The model under review builds one solid part; all positions refer to its coordinate system, in mm. A direction names the side the tool comes from. Round coordinates to 2 decimals unless told otherwise and drop trailing zeros. Order: outer loops, then holes, each group sorted by start corner. A loop starts at its lowest first (then second) coordinate and runs counter-clockwise, first axis right, second up.
from build123d import *

# Parameters (mm, degrees)
F0_W     = 101.6
F0_H     = 101.6
F1_DEPTH = 101.6
F2_T     = -12.7
F3_W     = 12.7
F3_H     = 76.2
F4_DEPTH = 6.35
F5_R     = 2.54
F6_DEPTH = 95.885
F7_R     = 5.08


with BuildPart() as f1:
    # F0 (on Top) → F1 (new body)
    with BuildSketch(Plane.XY):
        Rectangle(F0_W, F0_H)
    extrude(amount=F1_DEPTH)

    # F2
    f2_openings = [f1.faces().sort_by_distance(p)[0] for p in [
        (0, 0, 101.6),
    ]]
    offset(amount=F2_T, openings=f2_openings)

    # F3 (on face) → F4 (join)
    with BuildSketch(Plane.XY.offset(101.6)):
        with Locations((44.45, 0)):
            Rectangle(F3_W, F3_H)
    extrude(amount=F4_DEPTH)

    # F5 (on face) → F6 (cut)
    with BuildSketch(Plane.XZ.offset(38.1)):
        with Locations((44.505034, 104.681725)):
            Circle(F5_R)
    extrude(amount=-F6_DEPTH, mode=Mode.SUBTRACT)

    # F7
    f7_edges = [f1.edges().sort_by_distance(p)[0] for p in [
        (38.1, 0, 107.95),
    ]]
    fillet(f7_edges, radius=F7_R)


solid = f1.part
(1) We need section C-C (y = -21). Give the boundary of the cut face in (x, z).
(2) We need section A-A (z = 26). Give the boundary of the cut face in (x, y), and give its area (3 significant figures).
(3) Tool access review of faces 4 (the flat face through (-50.8, -1, 50)), 5 (the flat face through (-38.1, -1, 57)), 6 (the flat face through (47.2, -38.1, 104.7)): name each direction out of +Z, -Z, +X, -X, +Y, -Y from which nothing blocks a thin tool from reaching the whole face with its end or side.
(4) We need section B-B (x = 25). Give the boundary of the cut face in (y, z).
(5) We need section D-D (x = -42). Give the boundary of the cut face in (y, z).
(6) The part is to be moulded in two halves that separate along Y. For faces 1 (the flat face through (-1, -38.1, 57)), 2 (the cylindrical face through (43.954, -0.533, 102.202)), 3 (the flat face through (47.2, 38.1, 104.7)), say which applies: pulls with the +Y half, pulls with the -Y half, needs draft (parallel to the pull), parting line crosses it, or undercut.
(7) To check wall thickness, follow L1, parallel to Y at x = 5.5, z = 56.5; L2, parallel to Z at x = -42, y = 29. State the ranges of each line that lie inside material, in increasing order.
(8) Clearance check with flat-ended pins moving along their axes: P1, Ø5, axis at x = 38.5, y = 7.5, coming from the +Z side; P2, Ø7, axis at x = 47, z = 106, coming from the -Y side; P3, Ø4, axis at x = -25.5, y = 7, coming from the -Z side; P4, Ø1.9, axis at x = 43.5, z = 105.5, coming from the +Y side. State where each tip first meets the part, or that it passes through.
Verdict:
1. outline: (-50.8, 0) - (50.8, 0) - (50.8, 107.95) - (43.18, 107.95) arc R5.08 ccw to (38.1, 102.87) - (38.1, 12.7) - (-38.1, 12.7) - (-38.1, 101.6) - (-50.8, 101.6) - close; hole circle Ø5.08 at (44.51, 104.68)
2. outline: (-50.8, -50.8) - (50.8, -50.8) - (50.8, 50.8) - (-50.8, 50.8) - close; hole (-38.1, -38.1) - (38.1, -38.1) - (38.1, 38.1) - (-38.1, 38.1) - close
2. area: 4,520 mm2
3. face 4: +Z, -Z, -X, +Y, -Y
3. face 5: +Z
3. face 6: +Z, +X, -X, -Y
4. outline: (-50.8, 0) - (50.8, 0) - (50.8, 101.6) - (38.1, 101.6) - (38.1, 12.7) - (-38.1, 12.7) - (-38.1, 101.6) - (-50.8, 101.6) - close
5. outline: (-50.8, 0) - (50.8, 0) - (50.8, 101.6) - (-50.8, 101.6) - close
6. face 1: undercut
6. face 2: needs draft
6. face 3: pulls with the +Y half
7. L1: y = -50.8 to -38.1, 38.1 to 50.8
7. L2: z = 0 to 101.6
8. P1: stops at z = 107.46
8. P2: stops at y = -38.1
8. P3: stops at z = 0
8. P4: passes through
